Check sheet for the modelled part. Datum: model origin and axes. Units: mm. Face numbers are marked on the shaded views. A direction names the side the tool comes from. Round coordinates to 2 decimals unless told otherwise and drop trailing zeros. Order: outer loops, then holes, each group sorted by start corner. A loop starts at its lowest first (then second) coordinate and runs counter-clockwise, first axis right, second up.
(1) Sectioned sample at B-B, the plane x = -88. Enter the section's corners in (y, z).
(2) Sectioned sample at C-C, the plane y = 0. Enter the section's corners in (x, z), and give its area (3 significant figures).
(3) Sectioned sample at D-D, the plane z = 25.5. Enter the section's corners in (x, y).
(4) Thickness scan on probe 1 along Z at (x, y) = (1, 0); probe 2 along Z at (x, y) = (-88, -30.3); probe 3 along X at (y, z) = (-30.9, 25.5). Record the ranges inside material, lowest first.
(5) Depth check by flat-ended pin: pin 1 (10 mm diameter, centred on x = -39.5, y = -24, fed in from -Z); pin 2 (3.5 mm diameter, centred on y = 0, z = 46, fed in from -X); pin 3 (6 mm diameter, centred on x = -2, z = -13, fed in from +Y). Enter the tip coordinate at first touch or a pass-through.
(6) Sectioned sample at A-A, the plane z = -26. Enter the section's corners in (x, y), and give its area (4 significant figures).
(7) Tool access check on the marked faces 1, 2 and 3. Record the directions out of +Z, -Z, +X, -X, +Y, -Y that give a thin tool (end or side, any length) a straight path to the whole face; none if there is none.
```python
from build123d import *

# Parameters (mm, degrees)
SKETCH_1_W               = 107.5
SKETCH_1_H               = 50
EXTRUDE_1_DEPTH          = 3
CHAMFER_1_SIZE           = 2
CUT_EXTRUDE_1_DEPTH      = 61.450909836
CUT_EXTRUDE_1_DEPTH_BACK = 61.450909836
SKETCH_3_R               = 1.5
CHAMFER_2_SIZE           = 0.5
SKETCH_4_W               = 20
SKETCH_4_H               = 1
EXTRUDE_2_DEPTH          = 3
EXTRUDE_3_DEPTH          = 3
EXTRUDE_4_DEPTH          = 20
SKETCH_7_R               = 1.5
CUT_EXTRUDE_2_DEPTH      = 30
SKETCH_8_W               = 70
SKETCH_8_H               = 47.5
CUT_EXTRUDE_3_DEPTH      = 10
CHAMFER_5_SIZE           = 2
CHAMFER_6_SIZE           = 2
CHAMFER_7_SIZE           = 2
SKETCH_9_W               = 3
SKETCH_9_H               = 81.75
EXTRUDE_5_DEPTH          = 4


with BuildPart() as part:
    # 草图1 → 凸台-拉伸1 (new body)
    with BuildSketch(Plane(origin=(0, 0, 0), x_dir=(0, 0, -1), z_dir=(1, 0, 0))):
        with Locations((0, -2.5)):
            Rectangle(SKETCH_1_W, SKETCH_1_H)
    extrude(amount=EXTRUDE_1_DEPTH)

    # 倒角1
    chamfer_1_edges = [part.edges().sort_by_distance(p)[0] for p in [
        (1.5, 22.5, 53.75),
        (1.5, 22.5, -53.75),
        (1.5, -27.5, -53.75),
        (1.5, -27.5, 53.75),
    ]]
    chamfer(chamfer_1_edges, length=CHAMFER_1_SIZE)

    # 草图3 → 切除-拉伸1 (cut, two sides: drawn at the far end of the back side and taken through both)
    with BuildSketch(Plane(origin=(3, 0, 0), x_dir=(0, 0, -1), z_dir=(1, 0, 0)).offset(-CUT_EXTRUDE_1_DEPTH_BACK)):
        with Locations((46, 0)):
            Circle(SKETCH_3_R)
        with Locations((-46, 0)):
            Circle(SKETCH_3_R)
    extrude(amount=CUT_EXTRUDE_1_DEPTH + CUT_EXTRUDE_1_DEPTH_BACK, mode=Mode.SUBTRACT)

    # 倒角2
    chamfer_2_edges = [part.edges().sort_by_distance(p)[0] for p in [
        (3, 0, -44.5),
        (3, 0, 47.5),
    ]]
    chamfer(chamfer_2_edges, length=CHAMFER_2_SIZE)


with BuildPart() as body_2:
    # 草图4 → 凸台-拉伸2 (new body)
    with BuildSketch(Plane(origin=(3, 0, 0), x_dir=(0, 0, -1), z_dir=(1, 0, 0))):
        with Locations((-40, -28)):
            Rectangle(SKETCH_4_W, SKETCH_4_H)
    extrude(amount=-EXTRUDE_2_DEPTH)

    # 草图5 → 凸台-拉伸3 (add)
    with BuildSketch(Plane.XZ.offset(28.5)):
        Polygon((3, 50), (3, 30), (-42, 30), (-42, -71), (-97, -71), (-97, 50), align=None)
    extrude(amount=EXTRUDE_3_DEPTH)

    # 草图6 → 凸台-拉伸4 (add)
    with BuildSketch(Plane(origin=(0, 0, 30), x_dir=(-1, 0, 0), z_dir=(0, 0, -1))):
        Polygon((0, -20.5), (8, -28.5), (0, -28.5), align=None)
    extrude(amount=-EXTRUDE_4_DEPTH)

    # 草图7 → 切除-拉伸2 (cut)
    with BuildSketch(Plane(origin=(0, -28.5, 0), x_dir=(1, 0, 0), z_dir=(0, 1, 0))):
        with Locations(Location((-88, 53.5, 0), (0, 0, 270))):
            Circle(SKETCH_7_R)
        with Locations(Location((-88, -25.5, 0), (0, 0, 270))):
            Circle(SKETCH_7_R)
    extrude(amount=-CUT_EXTRUDE_2_DEPTH, mode=Mode.SUBTRACT)


with BuildPart() as part_1:
    add(part.part)

    # Combine 1: union body 2
    add(body_2.part)

    # 草图8 → 切除-拉伸3 (cut)
    with BuildSketch(Plane(origin=(3, 0, 0), x_dir=(0, 0, -1), z_dir=(1, 0, 0))):
        with Locations((0, -1.25)):
            Rectangle(SKETCH_8_W, SKETCH_8_H)
    extrude(amount=-CUT_EXTRUDE_3_DEPTH, mode=Mode.SUBTRACT)

    # 倒角5
    chamfer_5_edges = [part_1.edges().sort_by_distance(p)[0] for p in [
        (-0.75, -25, 35),
        (1.5, -25, -35),
    ]]
    chamfer(chamfer_5_edges, length=CHAMFER_5_SIZE)

    # 倒角6
    chamfer_6_edges = [part_1.edges().sort_by_distance(p)[0] for p in [
        (1.5, 22.5, 35),
        (1.5, 22.5, -35),
    ]]
    chamfer(chamfer_6_edges, length=CHAMFER_6_SIZE)

    # 倒角7
    chamfer_7_edges = [part_1.edges().sort_by_distance(p)[0] for p in [
        (-42, -30, 30),
        (-97, -30, 50),
        (-97, -30, -71),
        (-42, -30, -71),
    ]]
    chamfer(chamfer_7_edges, length=CHAMFER_7_SIZE)

    # 草图9 → 凸台-拉伸5 (add)
    with BuildSketch(Plane.XZ.offset(27.5)):
        with Locations((1.5, -10.875)):
            Rectangle(SKETCH_9_W, SKETCH_9_H)
    extrude(amount=EXTRUDE_5_DEPTH)


solid = part_1.part
```
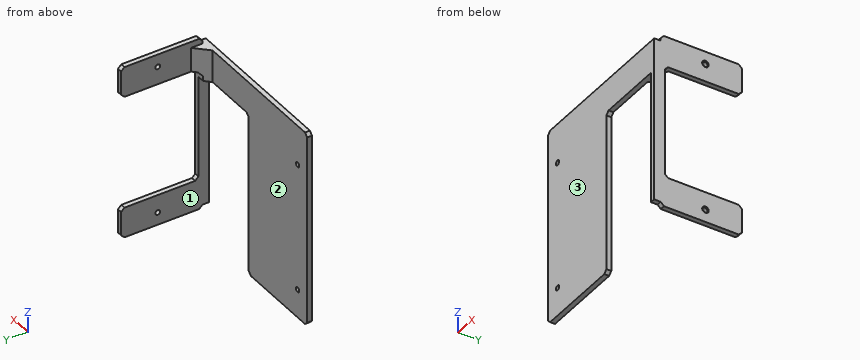
Derived:
1. outline: (-31.5, -71) - (-28.5, -71) - (-28.5, -55) - (-31.5, -55) - close; (-31.5, -52) - (-28.5, -52) - (-28.5, 24) - (-31.5, 24) - close; (-31.5, 27) - (-28.5, 27) - (-28.5, 50) - (-31.5, 50) - close
2. outline: (0, -53.75) - (3, -53.75) - (3, -48) - (2.5, -47.5) - (0, -47.5) - close; (0, -44.5) - (2.5, -44.5) - (3, -44) - (3, -35) - (0, -35) - close; (0, 35) - (3, 35) - (3, 44) - (2.5, 44.5) - (0, 44.5) - close; (0, 47.5) - (2.5, 47.5) - (3, 48) - (3, 53.75) - (0, 53.75) - close
2. area: 94.0 mm2
3. outline: (-97, -31.5) - (-89.5, -31.5) - (-89.5, -28.5) - (-97, -28.5) - close; (-86.5, -31.5) - (-42, -31.5) - (-42, -28.5) - (-86.5, -28.5) - close; (0, -31.5) - (3, -31.5) - (3, -25) - (0, -25) - close
4. probe 1: z = -53.75 to -47.5, -44.5 to -35, 35 to 44.5, 47.5 to 53.75
4. probe 2: z = -71 to -55, -52 to 24, 27 to 50
4. probe 3: x = -97 to -89.5, -86.5 to -42, 0 to 3
5. pin 1: stops at z = 28.32
5. pin 2: stops at x = 0
5. pin 3: stops at y = -25
6. outline: (-97, -31.5) - (-42, -31.5) - (-42, -28.5) - (-97, -28.5) - close; (0, -31.5) - (3, -31.5) - (3, -25) - (0, -25) - close
6. area: 184.5 mm2
7. face 1: -Z, +Y, -Y
7. face 2: +Z, -Z, -X, +Y
7. face 3: +Z, -Z, +X, -X, -Y
